```python
from build123d import *

# Parameters (mm, degrees)
F0_R      = 15
F1_DEPTH  = 25
F0_R_2    = 25
F1_FACE_R = 15
F2_DEPTH  = 5
F3_SIZE   = 2.54
F4_SIZE   = 2.54


with BuildPart() as f1:
    # F0 (on Top) → F1 (new body)
    with BuildSketch(Plane.XY):
        Circle(F0_R)
    extrude(amount=F1_DEPTH)

    # F0 (on Top) + F1_face (on face) → F2 (join)
    with BuildSketch(Plane.XY):
        Circle(F0_R_2)
        Circle(F0_R, mode=Mode.SUBTRACT)
    with BuildSketch(Plane.XY.offset(25)):
        Circle(F1_FACE_R)
    extrude(amount=F2_DEPTH)

    # F3
    f3_edges = [f1.edges().sort_by_distance(p)[0] for p in [
        (-25, 0, 0),
    ]]
    chamfer(f3_edges, length=F3_SIZE)

    # F4
    f4_edges = [f1.edges().sort_by_distance(p)[0] for p in [
        (-15, 0, 30),
    ]]
    chamfer(f4_edges, length=F4_SIZE)


solid = f1.part
```
Check sheet for the modelled part. Datum: model origin and axes. Units: mm. A direction names the side the tool comes from. Round coordinates to 2 decimals unless told otherwise and drop trailing zeros. Write each loop counter-clockwise with the first axis right and the second up, starting at its lowest first coordinate (ties: lowest second). Pieces come first, ordered by that corner, then holes. Notation, with made-up numbers: (-23, 81) -> (-5, 81) arc R23 ccw to (-5, 103) -> close; hole circle Ø10 at (-4, 34.5). An arc over 180 degrees is marked (long way). One line per question, with ' | ' between items. Start each with the question number.
1. Sectioned sample at A-A, the plane y = 0. Record the cut outline in (x, z).
2. Scan lines: line 1 along Z through (x, y) = (7, -17); line 2 along X through (y, z) = (-9.5, 23.5); line 3 along X through (y, z) = (5, 18.75). Record each from-to range of solid material in increasing order. Write a range as from..to.
3. Depth check by flat-ended pin: pin 1 (8 mm diameter, centred on x = 19.5, z = 14.5, fed in from +Y); pin 2 (8 mm diameter, centred on x = -0.5, y = -9, fed in from -Z); pin 3 (10 mm diameter, centred on y = -12, z = 18.5, fed in from -X); pin 4 (1.5 mm diameter, centred on y = 3, z = 19.5, fed in from -X). Enter the tip coordinate at first touch or a pass-through.
4. Sectioned sample at C-C, the plane z = 19.5. Record the cut outline in (x, y), then the cut area to 3 significant figures.
5. Set-up check for faces 1 (the face through (11, -11, 5)), 2 (the face through (0, 0, 30)): record each of +Z, -Z, +X, -X, +Y, -Y from which the full face is reachable in a straight line by a thin tool's end or side.
Taken from the geometry:
1) outline: (-25, 2.54) -> (-22.46, 0) -> (22.46, 0) -> (25, 2.54) -> (25, 5) -> (15, 5) -> (15, 27.46) -> (12.46, 30) -> (-12.46, 30) -> (-15, 27.46) -> (-15, 5) -> (-25, 5) -> close
2) line 1: z = 0..5 | line 2: x = -11.61..11.61 | line 3: x = -14.14..14.14
3) pin 1: passes through | pin 2: stops at z = 0 | pin 3: stops at x = -13.27 | pin 4: stops at x = -14.83
4) outline: circle Ø30 at (0, 0) | area: 707 mm^2
5) face 1: +Z | face 2: +Z, +X, -X, +Y, -Y
